Autodesk Inventor part; units mm, degrees
ref_plane "YZ Plane" through (0, 0, 0) normal (1, 0, 0) x (0, 1, 0)
ref_plane "XZ Plane" through (0, 0, 0) normal (0, 1, 0) x (-1, 0, 0)
ref_plane "XY Plane" through (0, 0, 0) normal (0, 0, 1) x (1, 0, 0)
sketch "Sketch1" plane through (0, 0, 0) normal (1, 0, 0) x (0, 1, 0)
  line L0 (0, 0) -> (107.95, 0)
  line L1 (107.95, 0) -> (107.95, -444.5)
  line L2 (107.95, -444.5) -> (0, -444.5)
  line L3 (0, -444.5) -> (0, 0)
  circle A0 centre (31.75, -50.8) radius 6.3627
  circle A1 centre (31.75, -393.7) radius 6.3627
  circle A2 centre (92.6338, -165.5318) radius 1.5875
  circle A3 centre (76.6318, -165.5318) radius 1.5875
  circle A4 centre (15.3162, -278.9682) radius 1.5875
  circle A5 centre (31.3182, -278.9682) radius 1.5875
  dimension "d0" = 107.95
  dimension "d1" = 444.5
  dimension "d2" = 12.7254
  dimension "d3" = 31.75
  dimension "d4" = 50.8
  dimension "d5" = 50.8
  dimension "d22" = 165.5318
  dimension "d23" = 3.175
  dimension "d24" = 15.3162
  dimension "d25" = 3.175
  dimension "d26" = 16.002
  dimension "d27" = 165.5318
  dimension "d28" = 3.175
  dimension "d29" = 15.3162
  dimension "d30" = 165.5318
  dimension "d31" = 3.175
  dimension "d32" = 16.002
  dimension "d33" = 165.5318
extrude "Extrusion1" add sketch "Sketch1" along normal blind 6.35 contours L0 L1 L2 L3 | A2 | A3 | A4 | A5
chamfer "Chamfer1" distance 38.1 angle 45 1 edges at (3.175, 0, 0)
chamfer "Chamfer2" distance 38.1 angle 45 1 edges at (3.175, 0, -444.5)
sketch "Sketch2" plane through (6.35, 0, 0) normal (1, 0, 0) x (0, 0, -1)
  line L0 (444.5, 38.1) -> (406.4, 0)
  line L1 (444.5, 38.1) -> (444.5, 107.95)
  line L2 (444.5, 107.95) -> (0, 107.95)
  line L3 (0, 107.95) -> (0, 38.1)
  line L4 (38.1, 0) -> (0, 38.1)
  line L5 (38.1, 0) -> (406.4, 0)
  circle A0 centre (393.7, 31.75) radius 6.3627
  circle A1 centre (50.8, 31.75) radius 6.3627
  circle A2 centre (120.4214, 77.9526) radius 6.3627
  circle A3 centre (324.0786, 29.9974) radius 6.3627
  point P0 (0, 0)
  dimension "d14" = 12.7254
  dimension "d15" = 120.4214
  dimension "d16" = 29.9974
  dimension "d17" = 12.7254
  dimension "d18" = 29.9974
  dimension "d19" = 120.4214
extrude "Extrusion2" cut sketch "Sketch2" against normal blind 25.4 contours A2 | A3
sketch "Sketch3" plane through (6.35, 0, 0) normal (1, 0, 0) x (0, 0, -1)
  circle A0 centre (120.4214, 77.9526) radius 6.3627
  circle A1 centre (324.0786, 29.9974) radius 6.3627
  line L0 (444.5, 38.1) -> (406.4, 0)
  line L1 (444.5, 38.1) -> (444.5, 107.95)
  line L2 (444.5, 107.95) -> (0, 107.95)
  line L3 (0, 107.95) -> (0, 38.1)
  line L4 (38.1, 0) -> (0, 38.1)
  line L5 (38.1, 0) -> (406.4, 0)
  circle A2 centre (393.7, 31.75) radius 6.3627
  circle A3 centre (50.8, 31.75) radius 6.3627
  circle A4 centre (165.5318, 99.949) radius 1.5875
  circle A5 centre (165.5318, 83.947) radius 1.5875
  circle A6 centre (278.9682, 22.86) radius 1.5875
  circle A7 centre (278.9682, 38.862) radius 1.5875
  point P0 (0, 0)
  dimension "d34" = 3.175
  dimension "d35" = 165.5318
  dimension "d36" = 8.001
  dimension "d37" = 3.175
  dimension "d38" = 16.002
  dimension "d39" = 3.175
  dimension "d40" = 3.175
  dimension "d41" = 22.86
  dimension "d42" = 16.002
  dimension "d43" = 165.5318
extrude "Extrusion3" cut sketch "Sketch3" against normal blind 25.4 contours A4 | A5 | A6 | A7
sketch "Sketch5" plane through (6.35, 0, 0) normal (1, 0, 0) x (0, 0, -1)
  circle A0 centre (278.9682, 22.86) radius 1.5875
  circle A1 centre (165.5318, 99.949) radius 1.5875
  circle A2 centre (165.5318, 83.947) radius 1.5875
  circle A3 centre (278.9682, 38.862) radius 1.5875
  circle A4 centre (120.4214, 77.9526) radius 6.3627
  circle A5 centre (324.0786, 29.9974) radius 6.3627
  line L0 (444.5, 38.1) -> (406.4, 0)
  line L1 (444.5, 38.1) -> (444.5, 107.95)
  line L2 (444.5, 107.95) -> (0, 107.95)
  line L3 (0, 107.95) -> (0, 38.1)
  line L4 (38.1, 0) -> (0, 38.1)
  line L5 (38.1, 0) -> (406.4, 0)
  circle A6 centre (393.7, 31.75) radius 6.3627
  circle A7 centre (50.8, 31.75) radius 6.3627
  circle A8 centre (23.0124, 105.5624) radius 1.9685
  circle A9 centre (23.0124, 88.1126) radius 1.9685
  circle A10 centre (421.5384, 105.5624) radius 1.9685
  circle A11 centre (421.5384, 88.1126) radius 1.9685
  point P0 (0, 0)
  dimension "d59" = 3.937
  dimension "d60" = 23.0124
  dimension "d61" = 2.3876
  dimension "d62" = 3.937
  dimension "d64" = 3.937
  dimension "d65" = 3.937
  dimension "d66" = 2.3876
  dimension "d68" = 22.9616
  dimension "d71" = 19.8374
  dimension "d72" = 19.8374
extrude "Extrusion5" cut sketch "Sketch5" against normal blind 25.4 contours A8 | A9 | A10 | A11
properties part number "DriveTrain3.0"
Model file for the job. Use its own axes, mm. Round coordinates to 2 decimals unless told otherwise and drop trailing zeros. Loops run counter-clockwise (first coordinate to the right, second up) from the corner with the lowest first, then second, coordinate; pieces in that order, holes last.
1. Band-saw the part on A-A, the plane z = -50.8. List the corners of the cut face in (x, y).
Check values:
outline: (0, 0) - (6.35, 0) - (6.35, 25.39) - (0, 25.39) - close; (0, 38.11) - (6.35, 38.11) - (6.35, 107.95) - (0, 107.95) - close
2. Wall check: probe 1 along Z at (x, y) = (5.5, 30); probe 2 along Z at (x, y) = (4, 31.75); probe 3 along Y at (x, z) = (6, -320). Give the ranges that are in metal, low to high.
Check values:
probe 1: z = -436.4 to -399.82, -387.58 to -330.44, -317.72 to -56.92, -44.68 to -8.1
probe 2: z = -438.15 to -400.06, -387.34 to -330.2, -317.96 to -57.16, -44.44 to -6.35
probe 3: y = 0 to 25.11, 34.88 to 107.95
3. Mould opens along Y. For faces 1 (the cylindrical face through (3.219, 30.277, -317.722)), 2 (the cylindrical face through (3.13, 30.37, -44.59)), 3 (the flat face through (6.35, 53, -219)), 4 (the flat face through (3.2, 19.3, -425.7)) say: +Y half, -Y half, draft (parallel to the pull), parting line (faces both ways), or undercut.
Check values:
face 1: undercut
face 2: undercut
face 3: draft
face 4: -Y half
4. Band-saw the part on B-B, the plane x = 4.75. Count the separate pieces of the cut face and the enclosed holes in it, and give its area (3 significant figures).
Check values:
separate pieces: 1
enclosed holes: 12
area: 45,900 mm2
5. Band-saw the part on C-C, the plane y = 8. List the corners of the cut face in (x, z), and give its area (3 significant figures).
Check values:
outline: (0, -414.4) - (6.35, -414.4) - (6.35, -30.1) - (0, -30.1) - close
area: 2,440 mm2
6. Drop flat-ended pins along their axis: P1, Ø2.5, axis at y = 88.11, z = -23.01, coming from the -X side; P2, Ø3, axis at x = 2.5, y = 25, coming from the -Z side; P3, Ø1.5, axis at x = 2, y = 12.5, coming from the -Z side. Give the stop position or say it passes through.
Check values:
P1: passes through
P2: stops at z = -432.9
P3: stops at z = -419.65
